Input: dimensioned drawing with shaded views. Units: mm. Origin: part minimum x, y, z. A direction names the side the tool comes from. Round coordinates to 2 decimals unless told otherwise and drop trailing zeros. Order: outer loops, then holes, each group sorted by start corner. A loop starts at its lowest first (then second) coordinate and runs counter-clockwise, first axis right, second up. Notation, with made-up numbers: M 6.5,22 L 40.5,22 A27 ccw 40.5,53 Z; hole C -4.75,53 d1. An arc over 180 degrees is marked long. Use one line per item in the form item = value. Start each with the question number.
Q1. Section A-A (y = 5). Return the cut outline in (x, z), plus the area to 3 significant figures.
Q2. Section B-B (z = 26). Return the cut outline in (x, y).
Q3. Section C-C (x = 25.25). Return the cut outline in (y, z), plus the area to 3 significant figures.
Q4. Material intervals for probe 1 along Z at (x, y) = (25.4, 5); probe 2 along Z at (x, y) = (16.25, 21.25); probe 3 along Y at (x, z) = (8, 36.4), sorted ascending.
Q5. Reachability of the marked faces 4 and 5 from +Z, -Z, +X, -X, +Y, -Y: full face, straight path, thin tool, end or side. Return the list, or none.
Q6. Section D-D (y = 12). Return the cut outline in (x, z).
Q7. Pull-direction query (Z, two-part tool) for the marked faces 1, 2 and 3; classes: pulls with the +Z half, pulls with the -Z half, needs draft (parallel to the pull), parting line crosses it, or undercut.
Q8. Contact query for flat-ended pins moving along their axis: pin 1 (1.4 mm diameter, centred on y = 12, z = 12, fed in from +X) (3 decimals); pin 2 (3 mm diameter, centred on y = 12, z = 26, fed in from -X). Output: stop coordinate, or through.
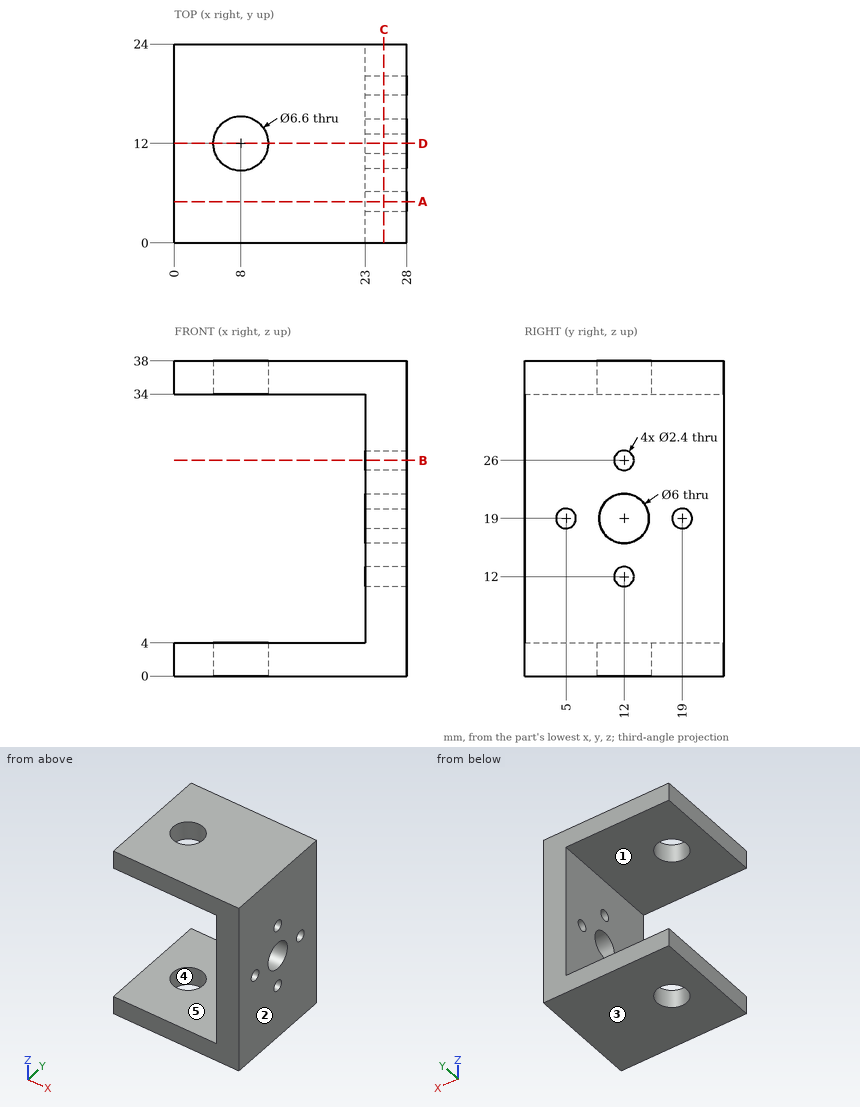
Results list:
q1.outline = M 0,0 L 28,0 L 28,17.8 L 23,17.8 L 23,4 L 0,4 Z; M 0,34 L 23,34 L 23,20.2 L 28,20.2 L 28,38 L 0,38 Z
q1.area = 362 mm2
q2.outline = M 23,0 L 28,0 L 28,10.8 L 23,10.8 Z; M 23,13.2 L 28,13.2 L 28,24 L 23,24 Z
q3.outline = M 0,0 L 24,0 L 24,38 L 0,38 Z; hole C 5,19 d2.4; hole C 12,19 d6; hole C 12,12 d2.4; hole C 12,26 d2.4; hole C 19,19 d2.4
q3.area = 866 mm2
q4.probe_1 = 0 to 17.8, 20.2 to 38
q4.probe_2 = 0 to 4, 34 to 38
q4.probe_3 = 0 to 8.7, 15.3 to 24
q5.face_4 = +Z, -Z
q5.face_5 = -X, +Y, -Y
q6.outline = M 0,0 L 4.7,0 L 4.7,4 L 0,4 Z; M 0,34 L 4.7,34 L 4.7,38 L 0,38 Z; M 11.3,0 L 28,0 L 28,10.8 L 23,10.8 L 23,4 L 11.3,4 Z; M 11.3,34 L 23,34 L 23,27.2 L 28,27.2 L 28,38 L 11.3,38 Z; M 23,13.2 L 28,13.2 L 28,16 L 23,16 Z; M 23,22 L 28,22 L 28,24.8 L 23,24.8 Z
q7.face_1 = undercut
q7.face_2 = needs draft
q7.face_3 = pulls with the -Z half
q8.pin_1 = through
q8.pin_2 = 23
